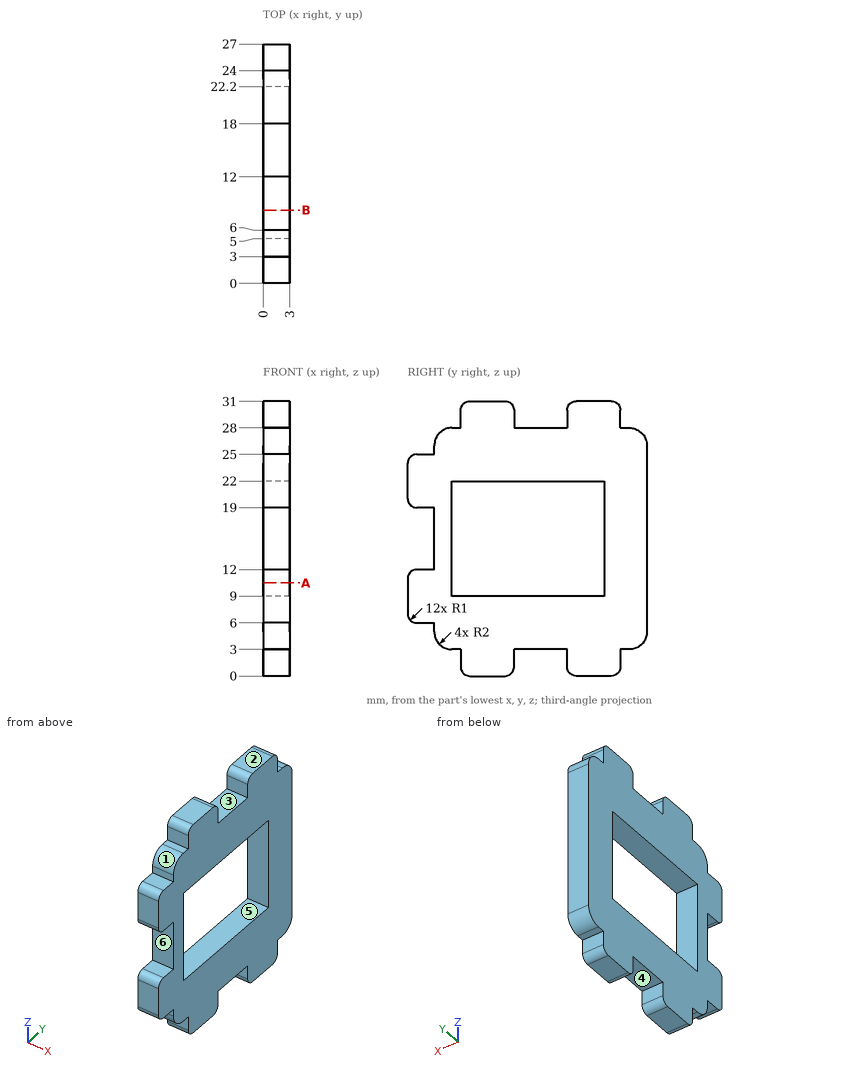
Geometry check sheet. Reference: drawing and pictorial views, mm from the part's lowest x, y, z. A direction names the side the tool comes from. Give positions to 0.01 mm unless a question says otherwise; leave off trailing zeros. Loops run counter-clockwise (first coordinate to the right, second up) from the corner with the lowest first, then second, coordinate; pieces in that order, holes last. Notation, with made-up numbers: (-17, 63.5) - (39, 63.5) arc R28 cw to (39, 86.5) - close; hole circle Ø4 at (-11, 43.25). An arc over 180 degrees is marked (long way). One line per question, with ' | ' between items. Start each with the question number.
1. Gauge pin test, flat ends, axial feed: pin 1 Ø0.5 at (x, y) = (2, 24.5) entering from +Z; pin 2 Ø1 at (x, y) = (1, 1.5) entering from +Z; pin 3 Ø0.6 at (x, z) = (2, 29) entering from +Y. Record the tip position at first contact, or that the pin passes through.
2. Draft check along Y on the marked faces 1, 2 and 3. Enter one of: released by +Y, released by -Y, zero draft, split by the parting line, or undercut.
3. Cross-section at A-A, the plane z = 10.5. Enter the section's corners in (x, y), plus the area to 3 significant figures.
4. Material ranges on line 1 along Z through (x, y) = (2.15, 12.5); line 2 along Y through (x, z) = (1.8, 16); line 3 along Z through (x, y) = (0.8, 7.5), recorded low to high. Write a range as [from, to].
5. Cross-section at B-B, the plane y = 8.25. Enter the section's corners in (x, z).
6. Set-up check for the marked faces 4, 5 and 6: record each of +Z, -Z, +X, -X, +Y, -Y from which the full face is reachable in a straight line by a thin tool's end or side.
Check result:
1) pin 1: stops at z = 28 | pin 2: stops at z = 25 | pin 3: stops at y = 24
2) face 1: released by -Y | face 2: zero draft | face 3: undercut
3) outline: (0, 0) - (3, 0) - (3, 5) - (0, 5) - close; (0, 22.2) - (3, 22.2) - (3, 27) - (0, 27) - close | area: 29.4 mm2
4) line 1: z = [3, 9], [22, 28] | line 2: y = [3, 5], [22.2, 27] | line 3: z = [0, 9], [22, 31]
5) outline: (0, 0) - (3, 0) - (3, 9) - (0, 9) - close; (0, 22) - (3, 22) - (3, 31) - (0, 31) - close
6) face 4: -Z, +X, -X | face 5: +X, -X | face 6: +X, -X, -Y
